```python
from build123d import *

# Parameters (mm, degrees)
F2_SIZE = 0.889
F3_SIZE = 0.381
F4_R    = 1.651


with BuildPart() as f1:
    # F0 (on Right) → F1 (revolve)
    with BuildSketch(Plane.YZ):
        with BuildLine():
            Line((0, 10.2108), (0, 4.024108))
            Line((0, 4.024108), (4.410164, 4.024108))
            Line((4.410164, 4.024108), (4.410164, 1.457856))
            Line((4.410164, 1.457856), (6.667502, 1.457856))
            Line((6.667502, 1.457856), (6.667502, 3.428277))
            ThreePointArc((6.667502, 3.428277), (8.527374, 7.918405), (13.017502, 9.778277))
            Line((13.017502, 9.778277), (76.3524, 9.778277))
            Line((76.3524, 9.778277), (87.180994, 6.057177))
            Line((87.180994, 6.057177), (100.203, 6.057177))
            Line((100.203, 6.057177), (100.203, 6.4897))
            Line((100.203, 6.4897), (87.180994, 6.4897))
            Line((87.180994, 6.4897), (76.3524, 10.2108))
            Line((76.3524, 10.2108), (6.667502, 10.2108))
            Line((6.667502, 10.2108), (4.299904, 8.636))
            Line((4.299904, 8.636), (2.159, 8.636))
            Line((2.159, 8.636), (2.159, 10.2108))
            Line((2.159, 10.2108), (0, 10.2108))
        make_face()
    revolve(axis=Axis((0, 1.0795, 0), (0, 1, 0)))

    # F2
    f2_edges = [f1.edges().sort_by_distance(p)[0] for p in [
        (0, 0, -10.2108),
    ]]
    chamfer(f2_edges, length=F2_SIZE)

    # F3
    f3_edges = [f1.edges().sort_by_distance(p)[0] for p in [
        (0, 0, -4.024108),
    ]]
    chamfer(f3_edges, length=F3_SIZE)

    # F4
    f4_edges = [f1.edges().sort_by_distance(p)[0] for p in [
        (0, 6.667502, -10.2108),
        (0, 4.299904, -8.636),
    ]]
    fillet(f4_edges, radius=F4_R)


solid = f1.part
```
Check sheet for the modelled part. Datum: model origin and axes. Units: mm. A direction names the side the tool comes from. Coordinates: 2 decimals unless noted, no trailing zeros. Loops run counter-clockwise (first coordinate to the right, second up) from the corner with the lowest first, then second, coordinate; pieces in that order, holes last. Notation, with made-up numbers: M -26,75 L 4,75 A15 ccw 4,94 Z; hole C 16.5,62 d4. An arc over 180 degrees is marked long. Answer as a JSON object with one key per item and string values.
1. Access from +Z, -Z, +X, -X, +Y, -Y to the whole of each face (thin tool, end or side, straight path). Record for faces 4 (the cylindrical face through (-3.686, 93.783, -4.807)), 5 (the cylindrical face through (2.937, 45.128, 9.327)), 6 (the cylindrical face through (3.07, 41.28, 9.74)), 7 (the cylindrical face through (3.393, 2.424, 2.163)).
Outcome:
{"face 4": "+Y", "face 5": "none", "face 6": "+Y, -Y", "face 7": "-Y"}
2. Release check for a two-part mould opening along Y. For faces 1 (the flat face through (0, 4.41, 2)), 2 (the cylindrical face through (2.59, 2.97, 8.24)), 3 (the cylindrical face through (3.07, 1.52, 9.74)) record: pulls with the +Y half, pulls with the -Y half, needs draft (parallel to the pull), parting line crosses it, or undercut.
Outcome:
{"face 1": "pulls with the -Y half", "face 2": "undercut", "face 3": "needs draft"}
3. Scan lines: L1, parallel to X at y = 96.75, z = 0; L2, parallel to Y at x = 0.75, z = -2.25; L3, parallel to X at y = 92, z = -3.25. Record each from-to range of solid material in increasing order. Write a range as from..to.
Outcome:
{"L1": "-6.49..-6.06, 6.06..6.49", "L2": "4.41..6.67", "L3": "-5.62..-5.11, 5.11..5.62"}
4. Depth check by flat-ended pin: P1, Ø4, axis at x = -0.5, z = -2, coming from the -Y side; P2, Ø6, axis at x = -4.5, y = 48.5, coming from the +Z side; P3, Ø5, axis at x = -3, z = 4.5, coming from the -Y side; P4, Ø10, axis at x = 0, z = -1, coming from the +Y side. Enter the tip coordinate at first touch or a pass-through.
Outcome:
{"P1": "y = 0.34", "P2": "z = 10.1", "P3": "y = 0", "P4": "y = 7.21"}
5. Sectioned sample at A-A on y = 28. Record the cut outline in (x, z), and give its area (3 significant figures).
Outcome:
{"outline": "C 0,0 d20.42; hole C 0,0 d19.56", "area": "27.2 mm²"}
